CAD build for the part. Positions are in the model's coordinates, mm. A direction names the side the tool comes from. Give positions to 0.01 mm unless a question says otherwise; leave off trailing zeros. Order: outer loops, then holes, each group sorted by start corner. A loop starts at its lowest first (then second) coordinate and runs counter-clockwise, first axis right, second up.
from build123d import *

# Parameters (mm, degrees)
F0_R          = 1.5
F0_R_2        = 2.6412895019
F1_DEPTH      = 20
F3_DEPTH      = 25
F3_DEPTH_BACK = 25
F6_R          = 3
F9_DEPTH      = 25
F11_W         = 149.615544593
F11_H         = 119.6888182312
F12_DEPTH     = 25


with BuildPart() as f1:
    # F0 (on Top) → F1 (new body)
    with BuildSketch(Plane.XY):
        with BuildLine():
            Line((-139.1577050821, 53.1693232265), (-48.1315898414, 53.1693232265))
            ThreePointArc((-48.1315898414, 53.1693232265), (-24.7040865671, 60.2304450376), (-48.9954501741, 63.1693232265))
            Line((-48.9954501741, 63.1693232265), (-139.1577050821, 63.1693232265))
            ThreePointArc((-139.1577050821, 63.1693232265), (-144.1577050821, 58.1693232265), (-139.1577050821, 53.1693232265))
        make_face()
        with Locations((-139.1577050821, 58.1693232265)):
            Circle(F0_R, mode=Mode.SUBTRACT)
        with BuildLine():
            ThreePointArc((-43.3736355328, 51.5244823211), (-44.7878490952, 51.5244823211), (-44.7878490952, 52.9386958835))
            Line((-44.7878490952, 52.9386958835), (-41.4003457692, 56.3261992095))
            ThreePointArc((-41.4003457692, 56.3261992095), (-39.9861322069, 56.3261992095), (-39.9861322069, 54.9119856471))
            Line((-39.9861322069, 54.9119856471), (-43.3736355328, 51.5244823211))
        make_face(mode=Mode.SUBTRACT)
        with BuildLine():
            ThreePointArc((-29.527561069, 52.9386958835), (-29.527561069, 51.5244823211), (-30.9417746314, 51.5244823211))
            Line((-30.9417746314, 51.5244823211), (-34.3292779574, 54.9119856471))
            ThreePointArc((-34.3292779574, 54.9119856471), (-34.3292779574, 56.3261992095), (-32.915064395, 56.3261992095))
            Line((-32.915064395, 56.3261992095), (-29.527561069, 52.9386958835))
        make_face(mode=Mode.SUBTRACT)
        with Locations((-37.1577050821, 59.1546263342)):
            Circle(F0_R_2, mode=Mode.SUBTRACT)
        with BuildLine():
            Line((-41.4003457692, 61.9830534589), (-44.7878490952, 65.3705567849))
            ThreePointArc((-44.7878490952, 65.3705567849), (-44.7878490952, 66.7847703473), (-43.3736355328, 66.7847703473))
            Line((-43.3736355328, 66.7847703473), (-39.9861322069, 63.3972670213))
            ThreePointArc((-39.9861322069, 63.3972670213), (-39.9861322069, 61.9830534589), (-41.4003457692, 61.9830534589))
        make_face(mode=Mode.SUBTRACT)
        with BuildLine():
            ThreePointArc((-30.9417746314, 66.7847703473), (-29.527561069, 66.7847703473), (-29.527561069, 65.3705567849))
            Line((-29.527561069, 65.3705567849), (-32.915064395, 61.983053459))
            ThreePointArc((-32.915064395, 61.9830534589), (-34.3292779574, 61.9830534589), (-34.3292779574, 63.3972670213))
            Line((-34.3292779574, 63.3972670213), (-30.9417746314, 66.7847703473))
        make_face(mode=Mode.SUBTRACT)
    extrude(amount=F1_DEPTH)

    # F2 (on face) → F3 (cut, two sides)
    with BuildSketch(Plane.XZ.offset(-53.1693232265)) as f3_sk:
        with BuildLine():
            add(Edge.make_bspline(
                [(-48.1315898414, 5.1997262053), (-55.5737955735, 5.517366778), (-70.0693075174, 9.5402547737), (-82.2478533544, 13.4277092293)],
                knots=[0, 0, 0, 0, 32.5655157772, 32.5655157772, 32.5655157772, 32.5655157772], degree=3))
            Line((-48.1315898414, 5.1997262053), (66.0970867342, 5.1997262053))
            Line((66.0970867342, 5.1997262053), (64.3360104363, 23.0218202323))
            Line((64.3360104363, 23.0218202323), (-14.16737711, 23.9689107984))
            Line((-14.16737711, 23.9689107984), (-21.0809869127, 20))
            Line((-21.0809869127, 20), (-48.1315898414, 24.3437178433))
            Line((-48.1315898414, 24.3437178433), (-48.1315898414, 13.4277092293))
            Line((-48.1315898414, 13.4277092293), (-82.2478533544, 13.4277092293))
        make_face()
    extrude(amount=-F3_DEPTH, mode=Mode.SUBTRACT)
    extrude(f3_sk.sketch, amount=F3_DEPTH_BACK, mode=Mode.SUBTRACT)

    # F7: sweep along a path in F4
    with BuildLine(Plane.XY.offset(5.1997262053)) as f7_path:
        Line((-61.2067505717, 58.1693232265), (-86.7135846391, 58.1693232265))
        Line((-86.7135846391, 58.1693232265), (-125.319480896, 58.1693232265))
        Line((-125.319480896, 58.1693232265), (-138.9607042074, 75.3938183188))
    # F6 (on face) → F7 (sweep, cut)
    with BuildSketch(Plane.YZ.offset(-48.1315898414)):
        with Locations((58.2011528313, 8.1997262053)):
            Circle(F6_R)
    sweep(path=f7_path.line, transition=Transition.RIGHT, mode=Mode.SUBTRACT)

    # F8 (on face) → F9 (cut)
    with BuildSketch(Plane.XZ.offset(-53.1693232265)):
        with BuildLine():
            add(Edge.make_bspline(
                [(-82.2478533544, 13.4277092293), (-114.2476946115, 13.955491595), (-135.7881426811, 12.4776158482), (-135.3534758091, 20)],
                knots=[0, 0, 0, 0, 53.5107666015, 53.5107666015, 53.5107666015, 53.5107666015], degree=3))
            Line((-82.2478533544, 13.4277092293), (-32.9686515033, 11.7128845304))
            Line((-32.9686515033, 11.7128845304), (-32.9686515033, 37.384595722))
            Line((-32.9686515033, 37.384595722), (-135.3534758091, 20))
        make_face()
    extrude(amount=-F9_DEPTH, mode=Mode.SUBTRACT)


with BuildPart() as f10_1:
    # F10: instance of F1
    add(f1.part.mirror(Plane.XZ))


with BuildPart() as f1_1:
    add(f1.part)

    # F11 (on face) → F12 (cut)
    with BuildSketch(Plane.XY.offset(20)):
        with Locations((-77.5791165652, 71.9989491627)):
            Rectangle(F11_W, F11_H)
    extrude(amount=-F12_DEPTH, mode=Mode.SUBTRACT)


solid = f10_1.part
1. Mould opens along Y. For faces 1 (the cylindrical face through (-144.156, -58.279, 9.86)), 2 (the flat face through (-72, -59, 0)), 3 (the flat face through (-41.7, -65.11, 2.56)), 4 (the flat face through (-103, -63.169, 5)) say: released by +Y, released by -Y, zero draft, split by the parting line, or undercut.
2. 3-axis set-ups, long thin cutter, end or side, ignore diameter. For faces 5 (the cylindrical face through (-130, -59.3, 8.1)), 6 (the flat face through (-37, -62, 5.2)), 7 (the flat face through (-41.7, -53.2, 2.6)), 8 (the cylindrical face through (-96.73, -57.811, 5.225)), 9 (the flat face through (-104, -53.169, 8)): which of +Z, -Z, +X, -X, +Y, -Y reach the whole face in a straight line?
3. Saw through at A-A on z = 3.75. Give the cut face in (x, y).
4. Pin check, flat tips, straight feed: P1, Ø1.5, axis at x = -118, y = -57, coming from the +Z side; P2, Ø1.5, axis at x = -85.5, z = 9, coming from the -Y side; P3, Ø3, axis at y = -50, z = 5.5, coming from the +X side. Stop position of each tip, or through.
5. Wall check: line 1 (X direction, y = -57.25, z = 1); line 2 (Z direction, x = -32, y = -58.5); line 3 (X direction, y = -59.5, z = 1.75). Give the ranges that are in metal, low to high.
Reported:
1. face 1: split by the parting line
1. face 2: zero draft
1. face 3: undercut
1. face 4: released by -Y
2. face 5: none
2. face 6: +Z, +X, +Y, -Y
2. face 7: +Z, -Z
2. face 8: +X
2. face 9: +Z, -Z, -X, +Y
3. outline: (-139.16, -63.17) - (-49, -63.17) arc R12.5 ccw (long way) to (-48.13, -53.17) - (-139.16, -53.17) arc R5 ccw to start; hole circle Ø3 at (-139.16, -58.17); hole (-44.79, -65.37) arc R1 ccw to (-43.37, -66.78) - (-39.99, -63.4) arc R1 ccw to (-41.4, -61.98) - close; hole (-44.79, -52.94) - (-41.4, -56.33) arc R1 ccw to (-39.99, -54.91) - (-43.37, -51.52) arc R1 ccw to start; hole circle Ø5.28 at (-37.16, -59.15); hole (-34.33, -63.4) - (-30.94, -66.78) arc R1 ccw to (-29.53, -65.37) - (-32.92, -61.98) arc R1 ccw to start; hole (-34.33, -54.91) arc R1 ccw to (-32.92, -56.33) - (-29.53, -52.94) arc R1 ccw to (-30.94, -51.52) - close
4. P1: stops at z = 13.96
4. P2: stops at y = -63.17
4. P3: stops at x = -27.3
5. line 1: x = -144.07 to -140.34, -137.97 to -38.99, -35.33 to -24.8
5. line 2: z = 0 to 5.2
5. line 3: x = -143.98 to -139.85, -138.47 to -39.78, -34.54 to -24.66
